Design review of the part built by this model. Coordinates are the model's own, in mm. A direction names the side the tool comes from. Give positions to 0.01 mm unless a question says otherwise; leave off trailing zeros. Order: outer loops, then holes, each group sorted by start corner. A loop starts at its lowest first (then second) coordinate and runs counter-clockwise, first axis right, second up. Notation, with made-up numbers: (-13.75, 43.5) -> (-7.75, 43.5) arc R12 ccw to (-7.75, 54.5) -> close; hole circle Ø6 at (-2, 25). An arc over 180 degrees is marked (long way). Return JSON: item names as keys, results as strings.
```python
from build123d import *

# Parameters (mm, degrees)
SKETCH_1_R      = 125
EXTRUDE_1_DEPTH = 30
SKETCH_4_R      = 60
EXTRUDE_2_DEPTH = 100
SKETCH_3_R      = 85


with BuildPart() as part:
    # ｽｹｯﾁ1 → ﾎﾞｽ - 押し出し1 (new body)
    with BuildSketch(Plane.XY):
        Circle(SKETCH_1_R)
    extrude(amount=EXTRUDE_1_DEPTH)

    # ｽｹｯﾁ3 → section 0 of loft_1
    with BuildSketch(Plane(origin=(0, 0, 70), x_dir=(-1, 0, 0), z_dir=(0, 0, -1)), mode=Mode.PRIVATE) as loft_1_s0:
        Circle(SKETCH_3_R)
    # loft up to a face of the part (loft_1)
    loft([loft_1_s0.sketch, Face(Wire([part.edges().sort_by_distance((-85.568388241, 91.121078428, 30))[0]]))])



with BuildPart() as body_2:
    # ｽｹｯﾁ4 → ﾎﾞｽ - 押し出し2 (new body)
    with BuildSketch(Plane(origin=(0, 0, 120), x_dir=(-1, 0, 0), z_dir=(0, 0, -1))):
        Circle(SKETCH_4_R)
    extrude(amount=-EXTRUDE_2_DEPTH)


with BuildPart() as part_1:
    add(part.part)

    add(body_2.part)  # loft_2 joins it to this body
    # loft from a face of the part (loft_2)
    loft([part_1.faces().sort_by_distance((0, 0, 70))[0], part_1.faces().sort_by_distance((0, 0, 120))[0]])


solid = part_1.part
```
Item 1: For pin 1 (10 mm diameter, centred on x = 97, y = 22, fed in from -Z); pin 2 (5 mm diameter, centred on x = -17, z = 107.5, fed in from +Y); pin 3 (2 mm diameter, centred on y = -53, z = 38, fed in from -X); pin 4 (1 mm diameter, centred on x = -78, y = 97, fed in from +Z), all flat-tipped, find the tip position at first contact; note any pin that passes through.
Result set:
{"pin 1": "stops at z = 0", "pin 2": "stops at y = 65.47", "pin 3": "stops at x = -105.53", "pin 4": "stops at z = 31.03"}
Item 2: Add section B-B (z = 166). Give the boundary of the cut face in (x, y), plus the area to 3 significant figures.
Result set:
{"outline": "circle Ø120 at (0, 0)", "area": "11,300 mm^2"}
Item 3: Wall thickness on L1, parallel to Y at x = 1, z = 137; L2, parallel to Y at x = 23, z = 54; L3, parallel to Z at x = -72, y = -0.5: over which ranges is each line inside the solid? List them lowest first. Write a range as [from, to].
Result set:
{"L1": "y = [-59.99, 59.99]", "L2": "y = [-98.35, 98.35]", "L3": "z = [0, 96]"}
Item 4: Machinability: for faces 1 (the face through (59.94, 2.64, 169.3)), 2 (the face through (1, 1, 220)), which of the approach directions +Z, -Z, +X, -X, +Y, -Y give a long, thin tool a straight path to every point of the face, cutting with its end or side? Answer none if there is none.
Result set:
{"face 1": "+Z", "face 2": "+Z, +X, -X, +Y, -Y"}
Item 5: Add section A-A (x = 0). Give the boundary of the cut face in (y, z).
Result set:
{"outline": "(-125, 0) -> (125, 0) -> (125, 30) -> (85, 70) -> (60, 120) -> (60, 220) -> (-60, 220) -> (-60, 120) -> (-85, 70) -> (-125, 30) -> close"}
Item 6: Add section C-C (z = 17). Give the boundary of the cut face in (x, y), plus the area to 3 significant figures.
Result set:
{"outline": "circle Ø250 at (0, 0)", "area": "49,100 mm^2"}
